Input: part model. Units: mm. Frame: model coordinates. Face numbers are marked on the shaded views. A direction names the side the tool comes from. Coordinates: 2 decimals unless noted, no trailing zeros. Write each loop counter-clockwise with the first axis right and the second up, starting at its lowest first coordinate (ties: lowest second). Pieces come first, ordered by that corner, then holes. Notation, with made-up numbers: (19.5, 58) - (57.5, 58) arc R24 ccw to (57.5, 81) - close; hole circle Ø3 at (79.25, 79.5). An arc over 180 degrees is marked (long way). Use a Markdown table: item, result. Add a question column.
Q1. Set-up query: the marked faces 1 and 2. Return all of +Z, -Z, +X, -X, +Y, -Y with unobstructed straight access to the full face (end or side cutting, diameter ignored); none if empty.
Q2. Pin query (flat end, axial travel): P1, Ø5, axis at x = 41, y = 0.5, coming from the -Z side. Return the tip coordinate at first contact, or that it passes through.
Q3. Material intervals for probe 1 along Y at (x, z) = (-38.1, 4); probe 2 along X at (y, z) = (3.5, 18); probe 3 along X at (y, z) = (5, 5.25), sorted ascending. Write a range as from..to.
Q4. Section query B-B (x = 0). Return the cut outline in (y, z), then the cut area to 3 significant figures.
Q5. Section query D-D (y = 1.5). Return the cut outline in (x, z).
Q6. Section query A-A (z = 2.5). Return the cut outline in (x, y).
Q7. Mould query, pull axis Y, two halves, no side actions, for the marked faces 3, 4 and 5. Classes: released by +Y, released by -Y, zero draft, split by the parting line, or undercut.
Q8. Section query C-C (x = -38.1). Return the cut outline in (y, z), then the cut area to 3 significant figures.
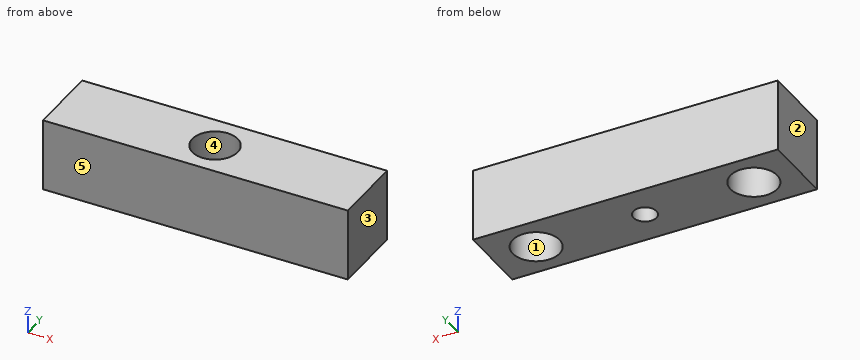
from build123d import *

# Parameters (mm, degrees)
SKETCH1_W                                            = 106.68
SKETCH1_H                                            = 25.4
BOSS_EXTRUDE1_DEPTH                                  = 25.4
SKETCH1_3_R                                          = 8.1915
CUT_EXTRUDE1_DEPTH                                   = 19.05
CBORE_FOR_1_4_BINDING_HEAD_MACHINE_SCREW_D           = 8.0264
CBORE_FOR_1_4_BINDING_HEAD_MACHINE_SCREW_CBORE_D     = 15.875
CBORE_FOR_1_4_BINDING_HEAD_MACHINE_SCREW_CBORE_DEPTH = 19.05


with BuildPart() as part:
    # Sketch1 → Boss-Extrude1 (new body)
    with BuildSketch(Plane.XY):
        Rectangle(SKETCH1_W, SKETCH1_H)
    extrude(amount=BOSS_EXTRUDE1_DEPTH)

    # Sketch1<3> → Cut-Extrude1 (cut)
    with BuildSketch(Plane.XY):
        with Locations(Location((-38.1, 0, 0), (0, 0, 180))):
            Circle(SKETCH1_3_R)
        with Locations(Location((38.1, 0, 0), (0, 0, 180))):
            Circle(SKETCH1_3_R)
    extrude(amount=CUT_EXTRUDE1_DEPTH, mode=Mode.SUBTRACT)

    # CBORE for 1/4 Binding Head Machine Screw1 (through all)
    with Locations(Plane.XY.offset(25.4)):
        with Locations((0, 0)):
            CounterBoreHole(CBORE_FOR_1_4_BINDING_HEAD_MACHINE_SCREW_D / 2, CBORE_FOR_1_4_BINDING_HEAD_MACHINE_SCREW_CBORE_D / 2, CBORE_FOR_1_4_BINDING_HEAD_MACHINE_SCREW_CBORE_DEPTH)


solid = part.part
Values follow:
| question | item | result |
|---|---|---|
| 1 | face 1 | -Z |
| 1 | face 2 | +Z, -Z, -X, +Y, -Y |
| 2 | P1 | z = 19.05 |
| 3 | probe 1 | -12.7..-8.19, 8.19..12.7 |
| 3 | probe 2 | -53.34..-45.51, -30.69..-7.12, 7.12..30.69, 45.51..53.34 |
| 3 | probe 3 | -53.34..-44.59, -31.61..31.61, 44.59..53.34 |
| 4 | outline | (-12.7, 0) - (-4.01, 0) - (-4.01, 6.35) - (-7.94, 6.35) - (-7.94, 25.4) - (-12.7, 25.4) - close; (4.01, 0) - (12.7, 0) - (12.7, 25.4) - (7.94, 25.4) - (7.94, 6.35) - (4.01, 6.35) - close |
| 4 | area | 292 mm2 |
| 5 | outline | (-53.34, 0) - (-46.15, 0) - (-46.15, 19.05) - (-30.05, 19.05) - (-30.05, 0) - (-3.72, 0) - (-3.72, 6.35) - (-7.79, 6.35) - (-7.79, 25.4) - (-53.34, 25.4) - close; (3.72, 0) - (30.05, 0) - (30.05, 19.05) - (46.15, 19.05) - (46.15, 0) - (53.34, 0) - (53.34, 25.4) - (7.79, 25.4) - (7.79, 6.35) - (3.72, 6.35) - close |
| 6 | outline | (-53.34, -12.7) - (53.34, -12.7) - (53.34, 12.7) - (-53.34, 12.7) - close; hole circle Ø16.38 at (-38.1, 0); hole circle Ø8.03 at (0, 0); hole circle Ø16.38 at (38.1, 0) |
| 7 | face 3 | zero draft |
| 7 | face 4 | undercut |
| 7 | face 5 | released by -Y |
| 8 | outline | (-12.7, 0) - (-8.19, 0) - (-8.19, 19.05) - (8.19, 19.05) - (8.19, 0) - (12.7, 0) - (12.7, 25.4) - (-12.7, 25.4) - close |
| 8 | area | 333 mm2 |
